Read the model definition and answer for the solid it produces. Units are mm, in the model's axes. Coordinates: 2 decimals unless noted, no trailing zeros. Order: outer loops, then holes, each group sorted by start corner. A loop starts at its lowest first (then second) coordinate and runs counter-clockwise, first axis right, second up.
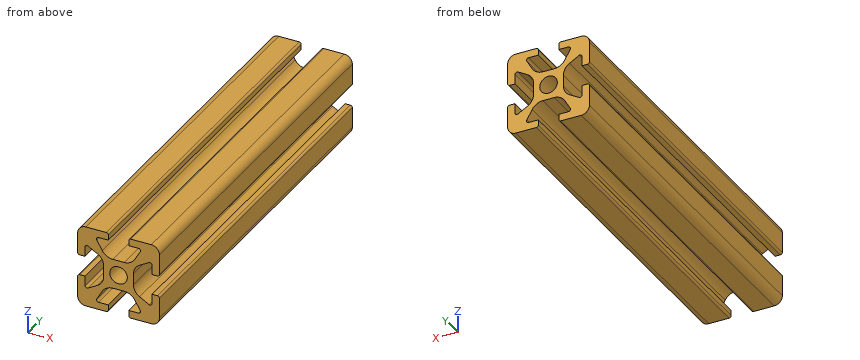
Solid Edge part; units mm, degrees
sketch "Sketch1" plane through (0, 0, 0) normal (0, -1, 0) x (1, 0, 0)
  line L0 (-10, -10) -> (10, -10)
  line L1 (10, -10) -> (10, 10)
  line L2 (10, 10) -> (-10, 10)
  line L3 (-10, 10) -> (-10, -10)
  dimension "D1" = 10
  dimension "D2" = 10
extrude "Protrusion1" add sketch "Sketch1" along normal mid plane 90
sketch "Sketch2" plane through (0, -45, 0) normal (0, -1, 0) x (1, 0, 0)
  line L0 (-2.5, 10) -> (-2.5, 8.2)
  line L1 (-2.5, 8.2) -> (-5.75, 8.2)
  line L2 (-5.75, 8.2) -> (-3.1231, 3.65)
  line L3 (-3.1231, 3.65) -> (3.1231, 3.65)
  line L4 (3.1231, 3.65) -> (5.75, 8.2)
  line L5 (5.75, 8.2) -> (2.5, 8.2)
  line L6 (2.5, 8.2) -> (2.5, 10)
  line L7 (2.5, 10) -> (-2.5, 10)
  dimension "D1" = 2.5
  dimension "D2" = 2.5
  dimension "D3" = 3.1231
extrude "Cutout1" cut sketch "Sketch2" against normal through all
fillet "Verrundung_1" radius 2 4 edges at (10, 0, 10) (-10, 0, 10) (10, 0, -10) (-10, 0, -10)
fillet "Verrundung_2" radius 3 2 edges at (-3.1231, 0, 3.65) (3.1231, 0, 3.65)
fillet "Verrundung_3" radius 0.5 4 edges at (-5.75, 0, 8.2) (5.75, 0, 8.2) (-2.5, 0, 10) (2.5, 0, 10)
hole "Bohrung_1" at (0, -45, 0) direction (0, 1, 0) diameter 4.3 end up to next
pattern_circular "Pattern1" count 4 over 360 about axis through (0, -45, 0) along (0, -1, 0) of "Cutout1"
fillet "Round1" radius 3 2 edges at (-3.65, 0, -3.1231) (-3.65, 0, 3.1231)
fillet "Round2" radius 0.5 4 edges at (-8.2, 0, -5.75) (-8.2, 0, 5.75) (-10, 0, -2.5) (-10, 0, 2.5)
fillet "Round3" radius 3 2 edges at (3.1231, 0, -3.65) (-3.1231, 0, -3.65)
fillet "Round4" radius 0.5 4 edges at (5.75, 0, -8.2) (-5.75, 0, -8.2) (2.5, 0, -10) (-2.5, 0, -10)
fillet "Round5" radius 3 2 edges at (3.65, 0, 3.1231) (3.65, 0, -3.1231)
fillet "Round6" radius 0.5 4 edges at (8.2, 0, 5.75) (8.2, 0, -5.75) (10, 0, 2.5) (10, 0, -2.5)
Q1. Straight lines are drawn through the part: L1, parallel to Z at x = 0, y = -4; L2, parallel to Z at x = -5, y = 17.5. For each, find the intervals that lie inside material, in ascending order.
Q2. Each of these flat-tipped pins is pushed along its axis until it touches: P1, Ø1.4, axis at y = -7.5, z = 0, coming from the -X side; P2, Ø4, axis at x = 0, z = 0, coming from the +Y side; P3, Ø2, axis at y = 15, z = -0.5, coming from the +X side; P4, Ø2, axis at x = -0.5, y = 7.5, coming from the +Z side. Where does it stop, or does it pass through?
Q3. The part is cut by section A-A, the plane x = 0. Determine the outline of the cut face in (y, z), then the cut area to 3 significant figures.
Q4. The part is cut by section B-B, the plane z = 0. Determine the outline of the cut face in (x, y), then the cut area to 3 significant figures.
Computed values:
1. L1: z = -3.65 to -2.15, 2.15 to 3.65
1. L2: z = -10 to -8.19, -6.9 to -3.9, 3.9 to 6.9, 8.19 to 10
2. P1: stops at x = -3.65
2. P2: passes through
2. P3: stops at x = 3.65
2. P4: stops at z = 3.65
3. outline: (-45, -3.65) - (45, -3.65) - (45, -2.15) - (-45, -2.15) - close; (-45, 2.15) - (45, 2.15) - (45, 3.65) - (-45, 3.65) - close
3. area: 270 mm2
4. outline: (-3.65, -45) - (-2.15, -45) - (-2.15, 45) - (-3.65, 45) - close; (2.15, -45) - (3.65, -45) - (3.65, 45) - (2.15, 45) - close
4. area: 270 mm2
